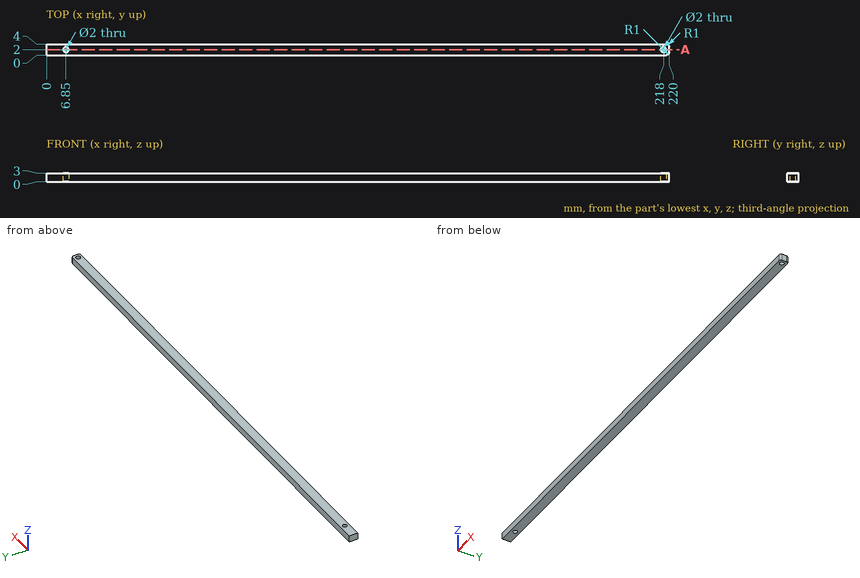
Can you work these out from the drawing? Everything is in mm from the part's minimum corner. Round coordinates to 2 decimals unless told otherwise and drop trailing zeros. Loops run counter-clockwise (first coordinate to the right, second up) from the corner with the lowest first, then second, coordinate; pieces in that order, holes last. Notation, with made-up numbers: (19.25, 1.25) - (27.25, 1.25) arc R19 ccw to (27.25, 19.25) - close; hole circle Ø7 at (-9, 44). An arc over 180 degrees is marked (long way). Answer as CSV lines item,"result".
1. I want a section at A-A on y = 2. List the corners of the cut face in (x, z) for me.
Filled in:
outline,"(0, 0) - (5.85, 0) - (5.85, 3) - (0, 3) - close; (7.85, 0) - (217, 0) - (217, 3) - (7.85, 3) - close; (219, 0) - (220, 0) - (220, 3) - (219, 3) - close"
2. For pin 1 Ø1.5 at (y, z) = (2, 2.5) entering from -X, with a flat end and sliding along its axis, tell me the tip position at first contact or that it passes through.
Filled in:
pin 1,"stops at x = 0"
3. Please list where these lines run through material, in increasing order: line 1 along X through (y, z) = (1.1, 1.05) (1 decimal); line 2 along X through (y, z) = (0.9, 2.15) (1 decimal); line 3 along X through (y, z) = (0.3, 1.9) (1 decimal). Write a range as [from, to].
Filled in:
line 1,"x = [0, 6.4], [7.3, 217.6], [218.4, 220]"
line 2,"x = [0, 220]"
line 3,"x = [0, 219.7]"
